from build123d import *

# Parameters (mm, degrees)
PAD_DEPTH    = 10
SKETCH001_W  = 30
SKETCH001_H  = 30
PAD001_DEPTH = 3
PAD002_DEPTH = 5


with BuildPart() as part:
    # Sketch → Pad (new body)
    with BuildSketch(Plane.XY):
        with BuildLine():
            Line((0, 0), (30, 0))
            ThreePointArc((30, 0), (54.07202, 18.385627), (35.736453, 42.495799))
            ThreePointArc((35.736453, 42.495799), (33.00775, 40.598561), (34.198631, 37.495799))
            ThreePointArc((31.598491, 5), (49.072145, 19.953776), (34.198631, 37.495799))
            Line((0, 5), (31.598491, 5))
            Line((0, 0), (0, 5))
        make_face()
    extrude(amount=PAD_DEPTH)

    # Sketch001 → Pad001 (join)
    with BuildSketch(Plane.YZ):
        with Locations((2.5, 5)):
            Rectangle(SKETCH001_W, SKETCH001_H)
    extrude(amount=-PAD001_DEPTH)

    # Sketch002 → Pad002 (join)
    with BuildSketch(Plane.XY.offset(2.5)):
        with BuildLine():
            ThreePointArc((0, 17.5), (19.159552, 9.062724), (39.948439, 6.593251))
            Line((39.948439, 6.593251), (35.370493, -0.035051))
            ThreePointArc((35.370493, -0.035051), (16.800197, -3.756112), (0, -12.5))
            Line((0, 17.5), (0, -12.5))
        make_face()
    extrude(amount=PAD002_DEPTH)


solid = part.part
Design review of the part built by this model. Coordinates are the model's own, in mm. A direction names the side the tool comes from. Coordinates: 2 decimals unless noted, no trailing zeros. Loops run counter-clockwise (first coordinate to the right, second up) from the corner with the lowest first, then second, coordinate; pieces in that order, holes last. Notation, with made-up numbers: (67, 57) -> (97, 57) arc R35 ccw to (97, 91) -> close; hole circle Ø7 at (70.25, 87). An arc over 180 degrees is marked (long way). Use a Markdown table: item, result. Add a question column.
Item 1: We need section C-C, the plane x = 8. Write out the cut boundary in (y, z), and give its area (3 significant figures).
Item 2: Machinability: for faces 5 (the flat face through (15, 0, 1)), 6 (the flat face through (16, 5, 1)), 7 (the flat face through (37, 5, 0)), 8 (the flat face through (15, 0, 9)), which of the approach directions +Z, -Z, +X, -X, +Y, -Y give a long, thin tool a straight path to every point of the face, cutting with its end or side? Answer none if there is none.
Item 3: We need section B-B, the plane y = 7.5. Write out the cut boundary in (x, z).
Item 4: We need section A-A, the plane x = 44.5. Write out the cut boundary in (y, z), and give its area (3 significant figures).
Item 5: The part is to be moulded in two halves that separate along X. For faces 1 (the flat face through (37, 5, 10)), 2 (the flat face through (16, 5, 9)), 3 (the flat face through (11, 9, 2.5)), 4 (the flat face through (-3, 2, 5)), say which applies: +X half, -X half, draft (parallel to the pull), parting line (faces both ways), or undercut.
Item 6: Clearance check with flat-ended pins moving along their axes: P1, Ø14, axis at x = 18.5, y = -4.5, coming from the -Z side; P2, Ø0.9, axis at x = -1, z = 3.5, coming from the +Y side; P3, Ø3, axis at x = 18, z = 1.5, coming from the -Y side; P4, Ø6, axis at x = 19.5, z = 13.5, coming from the +Y side. State where each tip first meets the part, or that it passes through.
Item 7: We need section D-D, the plane z = 5.5. Write out the cut boundary in (x, y).
Item 8: Wall thickness on L1, parallel to Z at x = 50.5, y = 19.5; L2, parallel to Z at x = 7.5, y = 10; L3, parallel to X at y = 14.5, z = -6: over which ranges is each line inside the solid? List them lowest first. Write a range as from..to.
Numbers:
| question | item | result |
|---|---|---|
| 1 | outline | (-7.58, 2.5) -> (0, 2.5) -> (0, 0) -> (5, 0) -> (5, 2.5) -> (13.14, 2.5) -> (13.14, 7.5) -> (5, 7.5) -> (5, 10) -> (0, 10) -> (0, 7.5) -> (-7.58, 7.5) -> close |
| 1 | area | 129 mm^2 |
| 2 | face 5 | -Z, -Y |
| 2 | face 6 | -Z, +Y |
| 2 | face 7 | -Z, +X, +Y, -Y |
| 2 | face 8 | +Z, -Y |
| 3 | outline | (-3, -10) -> (0, -10) -> (0, 2.5) -> (26.32, 2.5) -> (26.32, 7.5) -> (0, 7.5) -> (0, 20) -> (-3, 20) -> close; (41.57, 0) -> (49.27, 0) -> (49.27, 10) -> (41.57, 10) -> close |
| 4 | outline | (3.27, 0) -> (9.88, 0) -> (9.88, 10) -> (3.27, 10) -> close; (32.63, 0) -> (39.24, 0) -> (39.24, 10) -> (32.63, 10) -> close |
| 4 | area | 132 mm^2 |
| 5 | face 1 | draft |
| 5 | face 2 | undercut |
| 5 | face 3 | undercut |
| 5 | face 4 | -X half |
| 6 | P1 | stops at z = 0 |
| 6 | P2 | stops at y = 17.5 |
| 6 | P3 | stops at y = -3.73 |
| 6 | P4 | passes through |
| 7 | outline | (-3, -12.5) -> (0, -12.5) arc R67.35 cw to (33.35, -0.18) arc R21.44 ccw to (35.74, 42.5) arc R2.69 ccw to (34.2, 37.5) arc R16.3 cw to (39.95, 6.59) arc R70.85 cw to (0, 17.5) -> (-3, 17.5) -> close |
| 8 | L1 | z = 0..10 |
| 8 | L2 | z = 2.5..7.5 |
| 8 | L3 | x = -3..0 |
